Check sheet for the modelled part. Datum: model origin and axes. Units: mm. A direction names the side the tool comes from. Give positions to 0.01 mm unless a question says otherwise; leave off trailing zeros. Order: outer loops, then holes, each group sorted by start corner. A loop starts at its lowest first (then second) coordinate and runs counter-clockwise, first axis right, second up. Notation, with made-up numbers: (83.5, 32.25) -> (117.5, 32.25) arc R9 ccw to (117.5, 47.25) -> close; hole circle Ø9 at (59.5, 37.25). An arc over 180 degrees is marked (long way). Write each question's results on one line, items separated by ' | '.
from build123d import *

# Parameters (mm, degrees)
ESQUISSE1_R             = 15
EXTRUSION1_DEPTH        = 42
ESQUISSE2_OUTSIDE_W     = 43.94
ESQUISSE2_OUTSIDE_H     = 43.94
ESQUISSE2_OUTSIDE_R     = 13.5
ENL_V_MAT_EXTRU_1_DEPTH = 4
ESQUISSE3_OUTSIDE_W     = 43.94
ESQUISSE3_OUTSIDE_H     = 43.94
ESQUISSE3_OUTSIDE_R     = 13
ENL_V_MAT_EXTRU_2_DEPTH = 2
ESQUISSE4_OUTSIDE_W     = 43.94
ESQUISSE4_OUTSIDE_H     = 43.94
ESQUISSE4_OUTSIDE_R     = 13.75
ENL_V_MAT_EXTRU_3_DEPTH = 1
ESQUISSE5_OUTSIDE_W     = 43.94
ESQUISSE5_OUTSIDE_H     = 43.94
ESQUISSE5_OUTSIDE_R     = 14
ENL_V_MAT_EXTRU_4_DEPTH = 8
CHANFREIN1_SIZE         = 0.5
CHANFREIN2_SIZE         = 1.5
ESQUISSE6_R             = 5
EXTRUSION2_DEPTH        = 1.5
EXTRUSION3_START        = 2
ESQUISSE7_R             = 5
EXTRUSION3_DEPTH        = 2
ESQUISSE8_R             = 2.5
EXTRUSION4_DEPTH        = 0.9
EXTRUSION5_START        = 0.9
ESQUISSE9_R             = 2.5
EXTRUSION5_DEPTH        = 0.9
ENL_V_MAT_EXTRU_5_REACH = 53.839
ESQUISSE10_R            = 1.5
ESQUISSE11_R            = 2
ENL_V_MAT_EXTRU_6_DEPTH = 10
TROU_TARAUD_M21_D       = 1.6
TROU_TARAUD_M21_DEPTH   = 3.2
TROU_TARAUD_M21_TIP     = 0.480688495
TROU_TARAUD_M22_D       = 1.6
TROU_TARAUD_M22_DEPTH   = 2.2
TROU_TARAUD_M22_TIP     = 0.480688495
ESQUISSE16_R            = 0.75
EXTRUSION6_DEPTH        = 0.5


with BuildPart() as part:
    # Esquisse1 → Extrusion1 (new body)
    with BuildSketch(Plane(origin=(0, 0, 0), x_dir=(1, 0, 0), z_dir=(0, 1, 0))):
        with Locations(Location((0, 0, 0), (0, 0, 90))):
            Circle(ESQUISSE1_R)
    extrude(amount=EXTRUSION1_DEPTH)

    # Esquisse2 outside → Enlèv. mat.-Extru.1 (cut)
    with BuildSketch(Plane(origin=(0, 42, 0), x_dir=(1, 0, 0), z_dir=(0, 1, 0))):
        Rectangle(ESQUISSE2_OUTSIDE_W, ESQUISSE2_OUTSIDE_H)
        with Locations(Location((0, 0, 0), (0, 0, 270))):
            Circle(ESQUISSE2_OUTSIDE_R, mode=Mode.SUBTRACT)
    extrude(amount=-ENL_V_MAT_EXTRU_1_DEPTH, mode=Mode.SUBTRACT)

    # Esquisse3 outside → Enlèv. mat.-Extru.2 (cut)
    with BuildSketch(Plane.XZ):
        Rectangle(ESQUISSE3_OUTSIDE_W, ESQUISSE3_OUTSIDE_H)
        with Locations(Location((0, 0, 0), (0, 0, 270))):
            Circle(ESQUISSE3_OUTSIDE_R, mode=Mode.SUBTRACT)
    extrude(amount=-ENL_V_MAT_EXTRU_2_DEPTH, mode=Mode.SUBTRACT)

    # Esquisse4 outside → Enlèv. mat.-Extru.3 (cut)
    with BuildSketch(Plane.XZ.offset(-2)):
        Rectangle(ESQUISSE4_OUTSIDE_W, ESQUISSE4_OUTSIDE_H)
        with Locations(Location((0, 0, 0), (0, 0, 270))):
            Circle(ESQUISSE4_OUTSIDE_R, mode=Mode.SUBTRACT)
    extrude(amount=-ENL_V_MAT_EXTRU_3_DEPTH, mode=Mode.SUBTRACT)

    # Esquisse5 outside → Enlèv. mat.-Extru.4 (cut)
    with BuildSketch(Plane.XZ.offset(-3)):
        Rectangle(ESQUISSE5_OUTSIDE_W, ESQUISSE5_OUTSIDE_H)
        with Locations(Location((0, 0, 0), (0, 0, 270))):
            Circle(ESQUISSE5_OUTSIDE_R, mode=Mode.SUBTRACT)
    extrude(amount=-ENL_V_MAT_EXTRU_4_DEPTH, mode=Mode.SUBTRACT)

    # Chanfrein1
    chanfrein1_edges = [part.edges().sort_by_distance(p)[0] for p in [
        (0, 42, -13.5),
    ]]
    chamfer(chanfrein1_edges, length=CHANFREIN1_SIZE)

    # Chanfrein2
    chanfrein2_edges = [part.edges().sort_by_distance(p)[0] for p in [
        (0, 38, -13.5),
    ]]
    chamfer(chanfrein2_edges, length=CHANFREIN2_SIZE - 0.0001)  # a hair under: the kernel refuses the full size

    # Esquisse6 → Extrusion2 (add)
    with BuildSketch(Plane(origin=(0, 42, 0), x_dir=(1, 0, 0), z_dir=(0, 1, 0))):
        with Locations(Location((0, 0, 0), (0, 0, 270))):
            Circle(ESQUISSE6_R)
    extrude(amount=EXTRUSION2_DEPTH)

    # Esquisse7 → Extrusion3 (add)
    with BuildSketch(Plane.XZ.offset(EXTRUSION3_START)):
        with Locations(Location((0, 0, 0), (0, 0, 90))):
            Circle(ESQUISSE7_R)
    extrude(amount=-EXTRUSION3_DEPTH)

    # Esquisse8 → Extrusion4 (add)
    with BuildSketch(Plane(origin=(0, 43.5, 0), x_dir=(1, 0, 0), z_dir=(0, 1, 0))):
        with Locations(Location((0, 0, 0), (0, 0, 270))):
            Circle(ESQUISSE8_R)
    extrude(amount=EXTRUSION4_DEPTH)

    # Esquisse9 → Extrusion5 (add)
    with BuildSketch(Plane.XZ.offset(2).offset(EXTRUSION5_START)):
        with Locations(Location((0, 0, 0), (0, 0, 90))):
            Circle(ESQUISSE9_R)
    extrude(amount=-EXTRUSION5_DEPTH)

    # Esquisse10 → Enlèv. mat.-Extru.5 (cut, up to next)
    with BuildSketch(Plane.XZ.offset(2.9), mode=Mode.PRIVATE) as enl_v_mat_extru_5_sk1:
        with Locations(Location((0, 0, 0), (0, 0, 270))):
            Circle(ESQUISSE10_R)
    enl_v_mat_extru_5_tool1 = extrude(enl_v_mat_extru_5_sk1.sketch, amount=-ENL_V_MAT_EXTRU_5_REACH, mode=Mode.PRIVATE) & part.part
    add(enl_v_mat_extru_5_tool1.solids().sort_by_distance((0, -2.9, 0))[0], mode=Mode.SUBTRACT)

    # Esquisse11 → Enlèv. mat.-Extru.6 (cut)
    with BuildSketch(Plane(origin=(0, 44.4, 0), x_dir=(1, 0, 0), z_dir=(0, 1, 0))):
        with Locations(Location((0, 0, 0), (0, 0, 270))):
            Circle(ESQUISSE11_R)
    extrude(amount=-ENL_V_MAT_EXTRU_6_DEPTH, mode=Mode.SUBTRACT)

    # Trou taraudé M21
    with Locations(Plane(origin=(0, 42, 0), x_dir=(-1, 0, 0), z_dir=(0, 1, 0))):
        with Locations((0, 8.5), (-7.361215932, 4.25), (-7.361215932, -4.25), (0, -8.5), (7.361215932, -4.25), (7.361215932, 4.25)):
            Hole(TROU_TARAUD_M21_D / 2, depth=TROU_TARAUD_M21_DEPTH)
            with Locations((0, 0, -(TROU_TARAUD_M21_DEPTH + TROU_TARAUD_M21_TIP / 2))):  # 118° drill point
                Cone(0, TROU_TARAUD_M21_D / 2, TROU_TARAUD_M21_TIP, mode=Mode.SUBTRACT)

    # Trou taraudé M22
    with Locations(Plane.XZ):
        with Locations((10, 0), (-10, 0)):
            Hole(TROU_TARAUD_M22_D / 2, depth=TROU_TARAUD_M22_DEPTH)
            with Locations((0, 0, -(TROU_TARAUD_M22_DEPTH + TROU_TARAUD_M22_TIP / 2))):  # 118° drill point
                Cone(0, TROU_TARAUD_M22_D / 2, TROU_TARAUD_M22_TIP, mode=Mode.SUBTRACT)

    # Esquisse16 → Extrusion6 (add)
    # profile 1 of 4: a face of its own
    with BuildSketch(Plane.XZ):
        with BuildLine():
            Line((0, 9.5), (-3, 9.5))
            Line((-3, 9.5), (-3, 6.5))
            Line((-3, 6.5), (0, 6.5))
            ThreePointArc((0, 6.5), (1.5, 8), (0, 9.5))
        make_face()
        with Locations(Location((0, 8, 0), (0, 0, 270))):
            Circle(ESQUISSE16_R, mode=Mode.SUBTRACT)
    # profile 2 of 4: a face of its own
    with BuildSketch(Plane.XZ):
        with BuildLine():
            Line((-7, 9.55), (-7, 6.55))
            Line((-7, 6.55), (-19.65, 6.55))
            ThreePointArc((-19.65, 6.55), (-20.9, 7.8), (-19.65, 9.05))
            Line((-19.65, 9.05), (-13, 9.05))
            Line((-13, 9.05), (-13, 9.55))
            Line((-13, 9.55), (-7, 9.55))
        make_face()
    # profile 3 of 4: a face of its own
    with BuildSketch(Plane.XZ):
        with BuildLine():
            Line((-13, -9.55), (-7, -9.55))
            Line((-7, -9.55), (-7, -6.55))
            Line((-7, -6.55), (-19.65, -6.55))
            ThreePointArc((-19.65, -6.55), (-20.9, -7.8), (-19.65, -9.05))
            Line((-19.65, -9.05), (-13, -9.05))
            Line((-13, -9.05), (-13, -9.55))
        make_face()
    # profile 4 of 4: a face of its own
    with BuildSketch(Plane.XZ):
        with BuildLine():
            Line((-3, -9.5), (-3, -6.5))
            Line((-3, -6.5), (0, -6.5))
            ThreePointArc((0, -6.5), (1.5, -8), (0, -9.5))
            Line((0, -9.5), (-3, -9.5))
        make_face()
        with Locations(Location((0, -8, 0), (0, 0, 90))):
            Circle(ESQUISSE16_R, mode=Mode.SUBTRACT)
    extrude(amount=EXTRUSION6_DEPTH)


solid = part.part
1. Gauge pin test, flat ends, axial feed: pin 1 Ø3 at (y, z) = (15.5, -11) entering from -X; pin 2 Ø1 at (y, z) = (10, -11.5) entering from -X; pin 3 Ø1.4 at (x, z) = (0, 8.5) entering from -Y. Record the tip position at first contact, or that the pin passes through.
Verdict:
pin 1: stops at x = -11.61 | pin 2: stops at x = -8.66 | pin 3: stops at y = -0.5
2. Section check A-A on x = -17. Record the cut outline in (y, z).
Verdict:
outline: (-0.5, -9.05) -> (0, -9.05) -> (0, -6.55) -> (-0.5, -6.55) -> close; (-0.5, 6.55) -> (0, 6.55) -> (0, 9.05) -> (-0.5, 9.05) -> close
3. Material ranges on probe 1 along X at (y, z) = (41.15, -4.25); probe 2 along X at (y, z) = (-0.15, -8); probe 3 along Y at (x, z) = (-12, -3.75), recorded low to high. Write a range as from..to.
Verdict:
probe 1: x = -12.81..-8.16, -6.56..6.56, 8.16..12.81 | probe 2: x = -20.88..-7, -3..-0.75, 0.75..1.5 | probe 3: y = 0..42
4. Section check B-B on y = 25. Record the cut outline in (x, z).
Verdict:
outline: circle Ø30 at (0, 0); hole circle Ø3 at (0, 0)
5. Section check C-C on y = 6. Record the cut outline in (x, z), then the cut area to 3 significant figures.
Verdict:
outline: circle Ø28 at (0, 0); hole circle Ø3 at (0, 0) | area: 609 mm^2
6. Mould release check, pull along X, two halves, no side actions. Record for faces 4 (the conical face through (9.861, 2.597, 0.006)), 5 (the flat face through (5, 2, -12.2)), 6 (the cylindrical face through (-7.91, 0.986, 10.316)): +X half, -X half, draft (parallel to the pull), parting line (faces both ways), or undercut.
Verdict:
face 4: undercut | face 5: draft | face 6: parting line
7. Access from +Z, -Z, +X, -X, +Y, -Y to the whole of each face (thin tool, end or side, straight path). Record for faces 1 (the cylindrical face through (-4.88, 42.74, -1.08)), 2 (the flat face through (-1, -0.5, 8)), 3 (the flat face through (-15, 0, 8)).
Verdict:
face 1: +Y | face 2: +Z, +X, -X, -Y | face 3: +Z, -X
